from build123d import *

# Parameters (mm, degrees)
F1_DEPTH = 63.5
F0_W     = 25.5134466434
F0_H     = 19.05
F2_DEPTH = 25.4
F3_DEPTH = 7.9375
F5_R     = 6.35


with BuildPart() as f1:
    # F0 (on Front) → F1 (new body, symmetric)
    with BuildSketch(Plane.XZ):
        Polygon((-41.275, -9.525), (41.275, -9.525), (41.275, 9.525), (22.225, 9.525), (-41.275, 9.525), align=None)
    extrude(amount=F1_DEPTH, both=True)

    # F0 (on Front) → F2 (join, symmetric)
    with BuildSketch(Plane.XZ):
        with BuildLine():
            Line((22.225, 9.525), (41.275, 9.525))
            Line((41.275, 9.525), (41.275, 12.7119745847))
            Line((41.275, 12.7119745847), (41.275, 27.0002))
            ThreePointArc((41.275, 27.0002), (45.9246798487, 38.2255201513), (57.15, 42.8752))
            Line((57.15, 42.8752), (60.325, 42.8752))
            Line((60.325, 42.8752), (60.325, 61.9252))
            Line((60.325, 61.9252), (57.15, 61.9252))
            add(Edge.make_bspline(
                [(54.0725699176, 61.7893513131), (55.1039994103, 61.839092438), (56.1300922565, 61.8842720565), (57.15, 61.9252)],
                knots=[108.8885339736, 108.8885339736, 108.8885339736, 108.8885339736, 111.5045361635, 111.5045361635, 111.5045361635, 111.5045361635], degree=3))
            ThreePointArc((54.0725699176, 61.7893513131), (31.3892268107, 50.5827823371), (22.225, 27.0002))
            Line((22.225, 27.0002), (22.225, 12.7119745847))
            Line((22.225, 12.7119745847), (22.225, 9.525))
        make_face()
        with Locations((73.0817233217, 52.4002)):
            Rectangle(F0_W, F0_H)
    extrude(amount=F2_DEPTH, both=True)

    # F0 (on Front) → F3 (join, symmetric)
    with BuildSketch(Plane.XZ):
        with BuildLine():
            add(Edge.make_bspline(
                [(-41.275, 9.525), (-41.0379751962, 49.7454198065), (11.1403255218, 59.7189256133), (54.0725699176, 61.7893513131)],
                knots=[0, 0, 0, 0, 108.8885339736, 108.8885339736, 108.8885339736, 108.8885339736], degree=3))
            Line((-41.275, 9.525), (22.225, 9.525))
            Line((22.225, 9.525), (22.225, 12.7119745847))
            Line((22.225, 12.7119745847), (22.225, 27.0002))
            ThreePointArc((22.225, 27.0002), (31.3892268107, 50.5827823371), (54.0725699176, 61.7893513131))
        make_face()
    extrude(amount=F3_DEPTH, both=True)

    # F0 (on Front) → F4 (revolve)
    with BuildSketch(Plane.XZ):
        Polygon((85.8384466434, 66.675), (85.8384466434, 61.9252), (85.8384466434, 42.8752), (85.8384466434, 38.1), (111.125, 38.1), (111.125, 66.675), align=None)
    revolve(axis=Axis((85.8384466434, 0, 52.3875), (0, 0, 1)))

    # F5
    f5_edges = [f1.edges().sort_by_distance(p)[0] for p in [
        (41.275, -63.5, 0),
        (-41.275, -63.5, 0),
        (-41.275, 63.5, 0),
        (41.275, 63.5, 0),
    ]]
    fillet(f5_edges, radius=F5_R)


solid = f1.part
Source: CAD feature listing. Evaluate the final solid. Frame: model axes, mm. A direction names the side the tool comes from. Coordinates: 2 decimals unless noted, no trailing zeros. Loops run counter-clockwise (first coordinate to the right, second up) from the corner with the lowest first, then second, coordinate; pieces in that order, holes last. Notation, with made-up numbers: (-16, 85.25) -> (42, 85.25) arc R25 ccw to (42, 114.25) -> close; hole circle Ø3 at (57, 80). An arc over 180 degrees is marked (long way). Answer in a Markdown table with one row per item. Add a question column.
Q1. Ray query, line 1 along Y through (x, z) = (7, 18); line 2 along Z through (x, y) = (-32, -13.5) (3 decimals); line 3 along X through (y, z) = (13.5, 21.5) (3 decimals). Return the intervals inside material, ascending.
Q2. Section A-A on z = -1.5. Return the cut outline in (x, y) (3 decimals).
Q3. Contact query for flat-ended pins moving along their axis: pin 1 Ø3 at (y, z) = (-13.5, 27.5) entering from +X; pin 2 Ø18.5 at (y, z) = (-24.5, 9) entering from +X (3 decimals); pin 3 Ø8 at (x, y) = (28.5, -20.5) entering from +Z. Output: stop coordinate, or through.
Q4. Pull-direction query (X, two-part tool) for faces 1 (the face through (-4, 7.938, 30)), 2 (the face through (45.8, -0.4, 38.1)), 3 (the face through (60, -2, 42.875)), 4 (the face through (22.225, 17, 18)); classes: pulls with the +X half, pulls with the -X half, needs draft (parallel to the pull), parting line crosses it, or undercut.
Q5. Section B-B on y = 41.5. Return the cut outline in (x, z) (3 decimals), and give its area (3 significant figures).
Q6. Reachability of faces 5 (the face through (31.635, 16.547, 50.849)), 6 (the face through (31.635, -16.791, 50.849)), 7 (the face through (86, 0, 38.1)) from +Z, -Z, +X, -X, +Y, -Y: full face, straight path, thin tool, end or side. Return the list, or none.
Computed values:
| question | item | result |
|---|---|---|
| 1 | line 1 | y = -7.94 to 7.94 |
| 1 | line 2 | z = -9.525 to 9.525 |
| 1 | line 3 | x = 22.225 to 41.275 |
| 2 | outline | (-41.275, -57.15) arc R6.35 ccw to (-34.925, -63.5) -> (34.925, -63.5) arc R6.35 ccw to (41.275, -57.15) -> (41.275, 57.15) arc R6.35 ccw to (34.925, 63.5) -> (-34.925, 63.5) arc R6.35 ccw to (-41.275, 57.15) -> close |
| 3 | pin 1 | stops at x = 41.4 |
| 3 | pin 2 | stops at x = 41.275 |
| 3 | pin 3 | stops at z = 51.74 |
| 4 | face 1 | needs draft |
| 4 | face 2 | undercut |
| 4 | face 3 | undercut |
| 4 | face 4 | pulls with the -X half |
| 5 | outline | (-41.275, -9.525) -> (41.275, -9.525) -> (41.275, 9.525) -> (-41.275, 9.525) -> close |
| 5 | area | 1,570 mm^2 |
| 6 | face 5 | +Z, -X, +Y |
| 6 | face 6 | +Z, -X, -Y |
| 6 | face 7 | -Z, +X, +Y, -Y |
